Part print with two shaded views. Sizes in mm from the minimum x, y, z corner. Give positions to 0.01 mm unless a question says otherwise; leave off trailing zeros. Write each loop counter-clockwise with the first axis right and the second up, starting at its lowest first coordinate (ties: lowest second). Pieces come first, ordered by that corner, then holes.
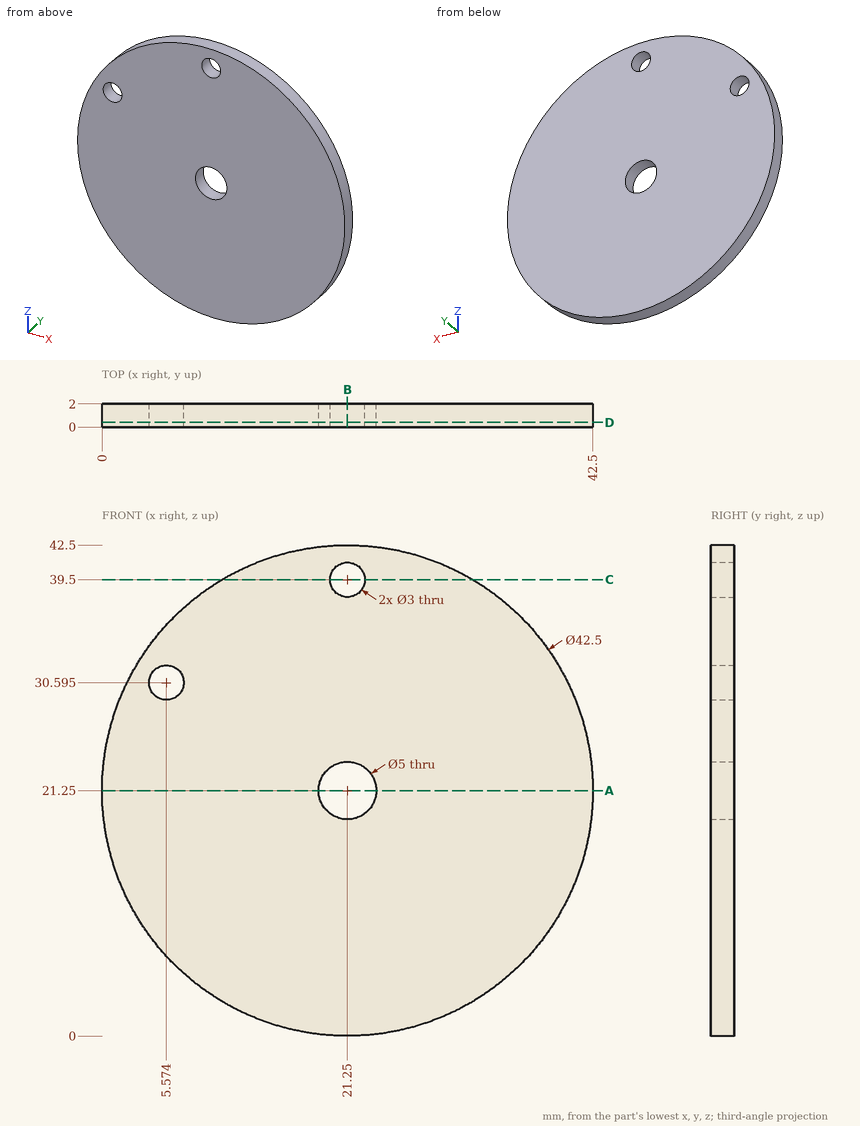
1) Saw through at C-C, the plane z = 39.5. Write the cut outline in (x, y).
Answers follow:
outline: (10.36, 0) - (19.75, 0) - (19.75, 2) - (10.36, 2) - close; (22.75, 0) - (32.14, 0) - (32.14, 2) - (22.75, 2) - close
2) Pin check, flat tips, straight feed: pin 1 Ø1.8 at (x, z) = (5.57, 30.59) entering from +Y; pin 2 Ø6.5 at (x, z) = (21.25, 21.25) entering from +Y. Stop position of each tip, or through.
Answers follow:
pin 1: passes through
pin 2: stops at y = 2
3) Saw through at D-D, the plane y = 0.4. Count the separate pieces of the cut face and the enclosed holes in it, then the cut area to 3 significant figures.
Answers follow:
separate pieces: 1
enclosed holes: 3
area: 1,380 mm2
4) Wall check: L1, parallel to Z at x = 21.25, y = 0.55; L2, parallel to Z at x = 22.5, y = 1.4 (1 decimal); L3, parallel to Z at x = 19, y = 0.9. Give the ranges that are in metal, low to high.
Answers follow:
L1: z = 0 to 18.75, 23.75 to 38, 41 to 42.5
L2: z = 0 to 19.1, 23.4 to 38.7, 40.3 to 42.5
L3: z = 0.12 to 20.16, 22.34 to 42.38
5) Saw through at B-B, the plane x = 21.25. Write the cut outline in (y, z).
Answers follow:
outline: (0, 0) - (2, 0) - (2, 18.75) - (0, 18.75) - close; (0, 23.75) - (2, 23.75) - (2, 38) - (0, 38) - close; (0, 41) - (2, 41) - (2, 42.5) - (0, 42.5) - close
6) Saw through at A-A, the plane z = 21.25. Write the cut outline in (x, y), then the cut area to 3 significant figures.
Answers follow:
outline: (0, 0) - (18.75, 0) - (18.75, 2) - (0, 2) - close; (23.75, 0) - (42.5, 0) - (42.5, 2) - (23.75, 2) - close
area: 75.0 mm2
